The drawing under review shows one solid part. Ordinate dimensions are in mm from its lowest x, y, z. A direction names the side the tool comes from. Round coordinates to 2 decimals unless told otherwise and drop trailing zeros. Write each loop counter-clockwise with the first axis right and the second up, starting at its lowest first coordinate (ties: lowest second). Pieces come first, ordered by that corner, then holes. Notation, with made-up numbers: M -38.75,32 L 13.25,32 A30 cw 13.25,71 Z; hole C 64,7.25 d7. An arc over 180 degrees is marked long. Write item = value, one per line. Start each with the question number.
Item 1: Take a section at C-C, the plane z = 17.25. Give the boundary of the cut face in (x, y), plus the area to 3 significant figures.
Item 2: For pin 1 Ø1.6 at (x, y) = (6, 6) entering from -Z; pin 2 Ø1.6 at (x, z) = (32, 22) entering from +Y; pin 3 Ø7 at (x, z) = (27.5, 12.5) entering from -Y; pin 4 Ø2.5 at (x, z) = (2, 12) entering from +Y, all flat-tipped, find the tip position at first contact; note any pin that passes through.
Item 3: Take a section at B-B, the plane y = 6. Give the boundary of the cut face in (x, z).
Item 4: Take a section at A-A, the plane x = 32. Give the boundary of the cut face in (y, z).
Item 5: The part is to be moulded in two halves that separate along X. For the marked faces 1, 2 and 3, say which applies: +X half, -X half, draft (parallel to the pull), parting line (faces both ways), or undercut.
Item 6: Take a section at D-D, the plane x = 20. Give the boundary of the cut face in (y, z).
Item 7: Tool access review of the marked faces 4, 5 and 6: name each direction out of +Z, -Z, +X, -X, +Y, -Y from which nothing blocks a thin tool from reaching the whole face with its end or side.
Item 8: To check wall thickness, follow line 1 along Z through (x, y) = (32, 6.1); line 2 along X through (y, z) = (6.35, 12); line 3 along X through (y, z) = (11.25, 7.25). State the ranges of each line that lie inside material, in increasing order.
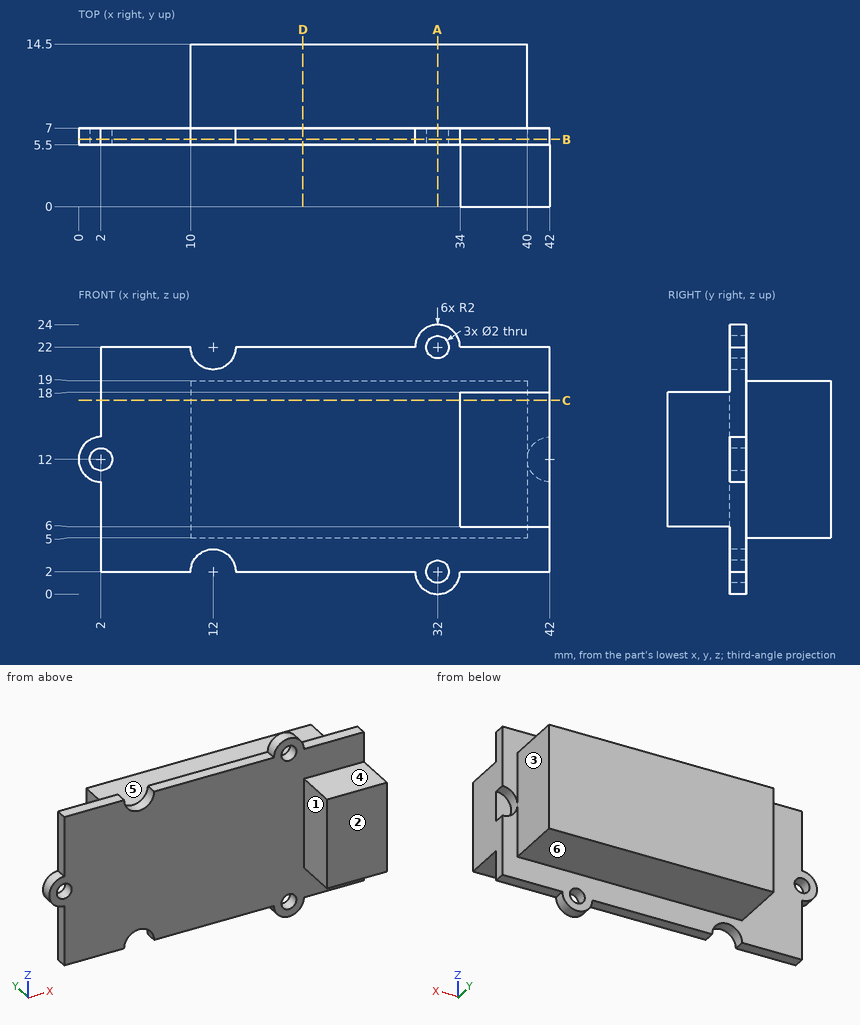
Response values:
q1.outline = M 2,5.5 L 34,5.5 L 34,0 L 42,0 L 42,7 L 40,7 L 40,14.5 L 10,14.5 L 10,7 L 2,7 Z
q1.area = 329 mm2
q2.pin_1 = 2
q2.pin_2 = through
q2.pin_3 = 5.5
q2.pin_4 = 7
q3.outline = M 2,2 L 10,2 A2 cw 14,2 L 30,2 A2 ccw 34,2 L 42,2 L 42,10 A2 cw 42,14 L 42,22 L 34,22 A2 ccw 30,22 L 14,22 A2 cw 10,22 L 2,22 L 2,14 A2 ccw 2,10 Z; hole C 2,12 d2; hole C 32,2 d2; hole C 32,22 d2
q4.outline = M 5.5,0 L 7,0 L 7,1 L 5.5,1 Z; M 5.5,3 L 7,3 L 7,5 L 14.5,5 L 14.5,19 L 7,19 L 7,21 L 5.5,21 Z; M 5.5,23 L 7,23 L 7,24 L 5.5,24 Z
q5.face_1 = -X half
q5.face_2 = draft
q5.face_3 = +X half
q6.outline = M 5.5,2 L 7,2 L 7,5 L 14.5,5 L 14.5,19 L 7,19 L 7,22 L 5.5,22 Z
q7.face_4 = +Z, +X, -X, -Y
q7.face_5 = +Z, +X, -X, +Y
q7.face_6 = -Z, +X, -X, +Y
q8.line_1 = 0 to 1, 3 to 21, 23 to 24
q8.line_2 = 0 to 1, 3 to 40
q8.line_3 = 10 to 40
